Answer from the drawing. Dimensions are ordinates in mm from the lowest x, y and z of the part. A direction names the side the tool comes from. Coordinates: 2 decimals unless noted, no trailing zeros. Write each loop counter-clockwise with the first axis right and the second up, starting at its lowest first coordinate (ties: lowest second). Pieces come first, ordered by that corner, then holes. Notation, with made-up numbers: (-34.75, -39.5) -> (-1.75, -39.5) arc R14 ccw to (-1.75, -32.5) -> close; hole circle Ø11 at (-30, -35). An arc over 180 degrees is marked (long way). Answer as a JSON object with one key per item and string values. Group by question number.
(1) Straight lines are drawn through the part: L1, parallel to Y at x = 4.5, z = 7; L2, parallel to Y at x = 13.5, z = 17.25; L3, parallel to X at y = 7.25, z = 5 (1 decimal). For each, find the intervals that lie inside material, in ascending order.
(2) Find section B-B (z = 16.5). Give the vertices of the cut face in (x, y).
(3) Which of the six approach directions +Z, -Z, +X, -X, +Y, -Y give full straight-line access (tool end or side, diameter ignored) to the marked faces 1, 2 and 3?
(4) Find section D-D (y = 17.5). Give the vertices of the cut face in (x, z).
(5) Find section C-C (y = 5.75). Give the vertices of the cut face in (x, z).
(6) Find section A-A (y = 11.25). Give the vertices of the cut face in (x, z) (1 decimal).
(7) Flat-ended cylindrical pins translate along their axes: P1, Ø5.5, axis at x = 9.5, z = 5, coming from the +Y side; P2, Ø1, axis at x = 15, z = 3, coming from the -Y side; P3, Ø8, axis at y = 8.5, z = 12, coming from the +X side; P4, Ø5, axis at x = 8, z = 15, coming from the -Y side. Find the tip coordinate at first contact, or state that the pin passes through.
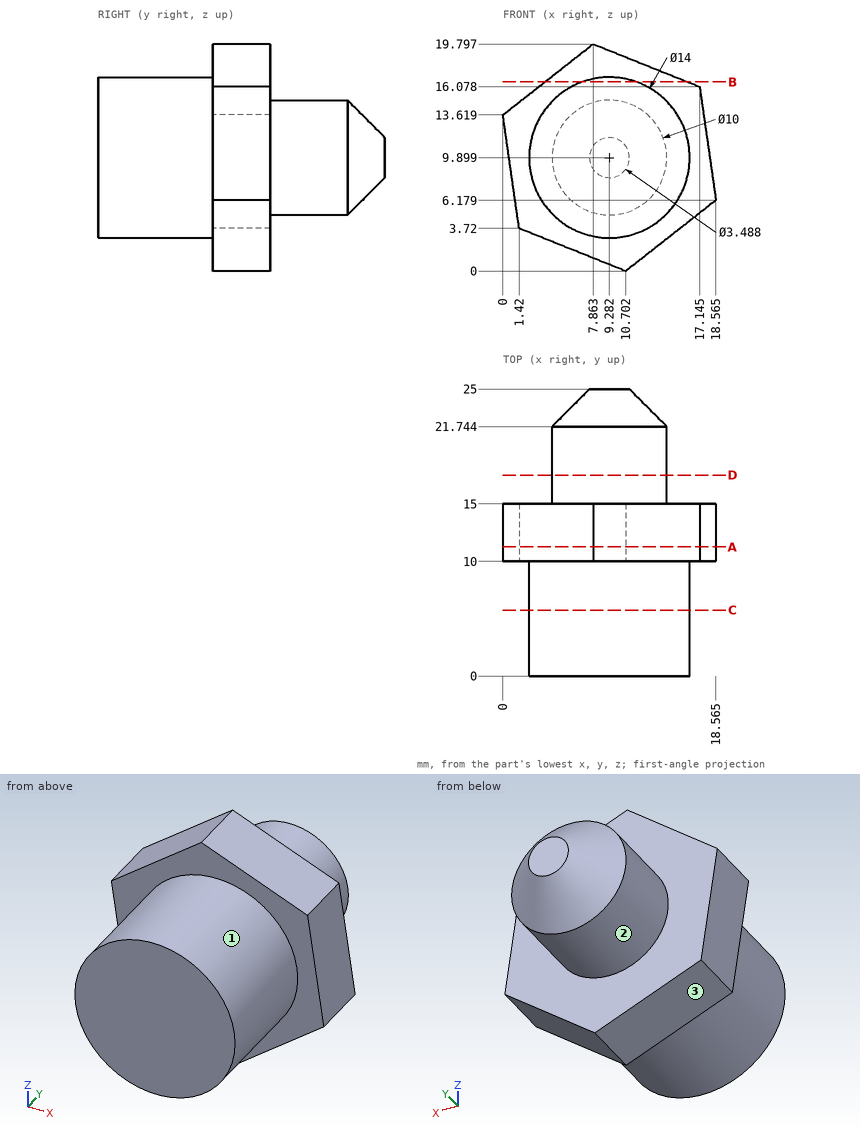
Results below:
{
 "1": {"L1": "y = 0 to 15", "L2": "y = 10 to 15", "L3": "x = 4.3 to 14.3"},
 "2": {"outline": "(3.67, 10) -> (6.95, 10) -> (6.95, 0) -> (11.61, 0) -> (11.61, 10) -> (16.09, 10) -> (16.09, 15) -> (3.67, 15) -> close"},
 "3": {"face 1": "-Y", "face 2": "+Y", "face 3": "-Z, -X, +Y, -Y"},
 "4": {"outline": "circle Ø10 at (9.28, 9.9)"},
 "5": {"outline": "circle Ø14 at (9.28, 9.9)"},
 "6": {"outline": "(0, 13.6) -> (1.4, 3.7) -> (10.7, 0) -> (18.6, 6.2) -> (17.1, 16.1) -> (7.9, 19.8) -> close"},
 "7": {"P1": "stops at y = 24.59", "P2": "stops at y = 10", "P3": "stops at x = 18.26", "P4": "stops at y = 0"}
}
